Input: dimensioned drawing with shaded views. Units: mm. Origin: part minimum x, y, z. A direction names the side the tool comes from. Coordinates: 2 decimals unless noted, no trailing zeros. Write each loop counter-clockwise with the first axis right and the second up, starting at its lowest first coordinate (ties: lowest second). Pieces come first, ordered by that corner, then holes. Notation, with made-up numbers: (-11, 37) - (46, 37) arc R23 cw to (46, 52) - close; hole circle Ø8 at (-1, 40). An arc over 180 degrees is marked (long way). One line per question, with ' | ' between items.
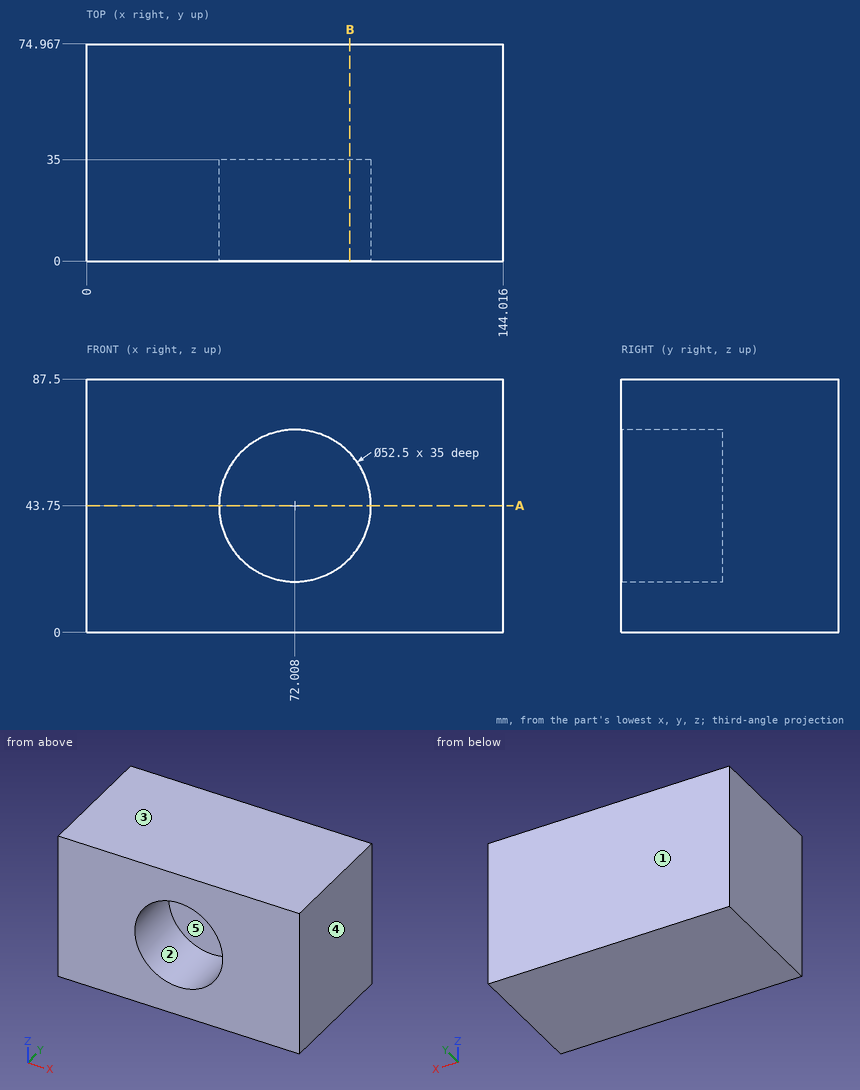
Item 1: Mould query, pull axis Z, two halves, no side actions, for the marked faces 3, 4 and 5. Classes: pulls with the +Z half, pulls with the -Z half, needs draft (parallel to the pull), parting line crosses it, or undercut.
Check sheet entries:
face 3: pulls with the +Z half | face 4: needs draft | face 5: undercut
Item 2: Cut plane A-A on z = 43.75. Return loops of the section in (x, y) (1 decimal), and give its area (3 significant figures).
Check sheet entries:
outline: (0, 0) - (45.8, 0) - (45.8, 35) - (98.3, 35) - (98.3, 0) - (144, 0) - (144, 75) - (0, 75) - close | area: 8,960 mm²
Item 3: Access query for the marked faces 1 and 2. Directions: +Z, -Z, +X, -X, +Y, -Y. A direction counts if a zero-diameter tool reaches every point of the face in a straight line with its end or side. Return the directions, or none.
Check sheet entries:
face 1: +Z, -Z, +X, -X, +Y | face 2: -Y
Item 4: Ray query, line 1 along X through (y, z) = (11, 43) (1 decimal); line 2 along X through (y, z) = (18.5, 44) (1 decimal); line 3 along Y through (x, z) = (67, 37.5). Return the intervals inside material, ascending. Write a range as [from, to].
Check sheet entries:
line 1: [0, 45.8], [98.2, 144] | line 2: [0, 45.8], [98.3, 144] | line 3: [35, 74.97]
Item 5: Cut plane B-B on x = 91. Return loops of the section in (y, z).
Check sheet entries:
outline: (0, 0) - (74.97, 0) - (74.97, 87.5) - (0, 87.5) - (0, 61.87) - (35, 61.87) - (35, 25.63) - (0, 25.63) - close
